```python
from build123d import *

# Parameters (mm, degrees)
PAD_DEPTH    = 4
SKETCH_W     = 23
SKETCH_H     = 4
POCKET_DEPTH = 5


with BuildPart() as part:
    # Sketch002 → Pad (new body)
    with BuildSketch(Plane.XY):
        with BuildLine():
            Line((65, 32.281557), (-10, 32.281557))
            ThreePointArc((-10, 32.281557), (-17.071068, 29.352625), (-20, 22.281557))
            Line((-20, 22.281557), (-20, 0))
            Line((-12.053457, 0), (-20, 0))
            Line((-12.053457, -4), (-12.053457, 0))
            Line((17.946543, -4), (-12.053457, -4))
            Line((17.946543, -4), (17.946543, 0))
            Line((27.946543, 0), (17.946543, 0))
            Line((27.946543, 0), (27.946543, 1))
            Line((27.946543, 1), (44.946543, 1))
            Line((44.946543, 1), (44.946543, 22.281557))
            ThreePointArc((49.946543, 27.281557), (46.411009, 25.817091), (44.946543, 22.281557))
            Line((49.946543, 27.281557), (65, 27.281557))
            Line((65, 27.281557), (65, 32.281557))
        make_face()
        with BuildLine():
            ThreePointArc((-6.164606, 24.307305), (-13.664606, 16.807305), (-6.164606, 9.307305))
            Line((-6.164606, 9.307305), (33.835394, 9.307305))
            ThreePointArc((33.835394, 9.307305), (41.335394, 16.807305), (33.835394, 24.307305))
            Line((33.835394, 24.307305), (-6.164606, 24.307305))
        make_face(mode=Mode.SUBTRACT)
    extrude(amount=PAD_DEPTH)

    # Sketch (on Face20 of Pad) → Pocket (cut)
    with BuildSketch(Plane.XY.offset(4)):
        with Locations((9.446543, 30.281557)):
            Rectangle(SKETCH_W, SKETCH_H)
    extrude(amount=-POCKET_DEPTH, mode=Mode.SUBTRACT)


solid = part.part
```
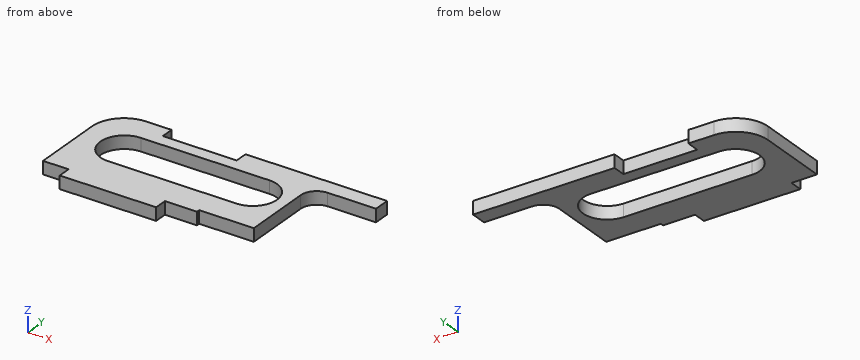
Design review of the part built by this model. Coordinates are the model's own, in mm. Give positions to 0.01 mm unless a question says otherwise; leave off trailing zeros. Write each loop counter-clockwise with the first axis right and the second up, starting at its lowest first coordinate (ties: lowest second). Pieces come first, ordered by that corner, then holes. Notation, with made-up numbers: (23.25, 49.5) - (62.25, 49.5) arc R32 ccw to (62.25, 78.5) - close; hole circle Ø4 at (-6, 1.25). An arc over 180 degrees is marked (long way). Return JSON: item names as keys, results as strings. Group by question number.
(1) To check wall thickness, follow probe 1 along Y at (x, z) = (20, 2.3); probe 2 along Y at (x, z) = (24, 1.7); probe 3 along X at (y, z) = (16.5, 0.5). State the ranges of each line that lie inside material, in increasing order.
(2) We need section A-A, the plane z = 1.3. Give the boundary of the cut face in (x, y).
(3) We need section B-B, the plane x = 10.5. Give the boundary of the cut face in (y, z), then the cut area to 3 significant figures.
(4) We need section D-D, the plane x = 52. Give the boundary of the cut face in (y, z).
(5) Insertion check: pin 1 (1.2 mm diameter, centred on x = 36.5, z = 1.5, fed in from -Y); pin 2 (2 mm diameter, centred on y = 10, z = 1.5, fed in from +X); pin 3 (2 mm diameter, centred on x = 12.5, z = 1, fed in from +Y). Each pin has a flat end and moves straight along its axis. Give the tip position at first contact, or say it passes through.
(6) We need section C-C, the plane y = 17. Give the boundary of the cut face in (x, z), then the cut area to 3 significant figures.
Reported:
{
 "1": {"probe 1": "y = 0 to 9.31, 24.31 to 28.28", "probe 2": "y = 0 to 9.31, 24.31 to 32.28", "probe 3": "x = -20 to -13.66, 41.33 to 44.95"},
 "2": {"outline": "(-20, 0) - (-12.05, 0) - (-12.05, -4) - (17.95, -4) - (17.95, 0) - (27.95, 0) - (27.95, 1) - (44.95, 1) - (44.95, 22.28) arc R5 cw to (49.95, 27.28) - (65, 27.28) - (65, 32.28) - (20.95, 32.28) - (20.95, 28.28) - (-2.05, 28.28) - (-2.05, 32.28) - (-10, 32.28) arc R10 ccw to (-20, 22.28) - close; hole (-6.16, 9.31) - (33.84, 9.31) arc R7.5 ccw to (33.84, 24.31) - (-6.16, 24.31) arc R7.5 ccw to start"},
 "3": {"outline": "(-4, 0) - (9.31, 0) - (9.31, 4) - (-4, 4) - close; (24.31, 0) - (28.28, 0) - (28.28, 4) - (24.31, 4) - close", "area": "69.1 mm2"},
 "4": {"outline": "(27.28, 0) - (32.28, 0) - (32.28, 4) - (27.28, 4) - close"},
 "5": {"pin 1": "stops at y = 1", "pin 2": "stops at x = 44.95", "pin 3": "stops at y = 28.28"},
 "6": {"outline": "(-20, 0) - (-13.66, 0) - (-13.66, 4) - (-20, 4) - close; (41.33, 0) - (44.95, 0) - (44.95, 4) - (41.33, 4) - close", "area": "39.8 mm2"}
}
